Design review of the part built by this model. Coordinates are the model's own, in mm. Face numbers are marked on the shaded views. A direction names the side the tool comes from. Coordinates: 2 decimals unless noted, no trailing zeros. Write each loop counter-clockwise with the first axis right and the second up, starting at its lowest first coordinate (ties: lowest second). Pieces come first, ordered by that corner, then holes. Notation, with made-up numbers: M 87.25,44 L 120.25,44 A19 cw 120.25,65 Z; hole C -38,52.25 d3. An arc over 180 degrees is marked long. Write item = value, one per line.
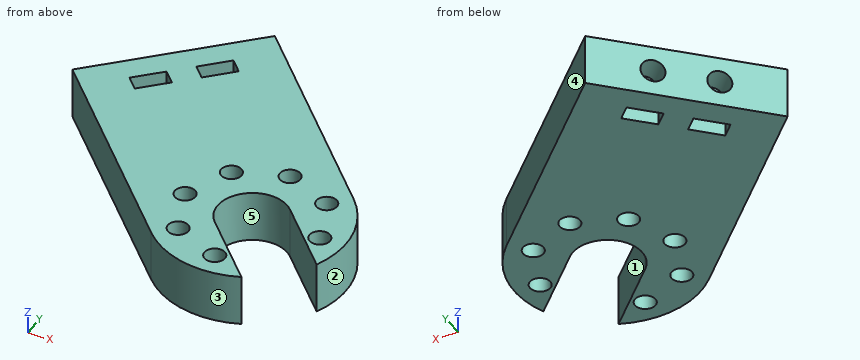
Autodesk Inventor part; units mm, degrees
ref_plane "YZ Plane" through (0, 0, 0) normal (1, 0, 0) x (0, 1, 0)
ref_plane "XZ Plane" through (0, 0, 0) normal (0, 1, 0) x (-1, 0, 0)
ref_plane "XY Plane" through (0, 0, 0) normal (0, 0, 1) x (1, 0, 0)
sketch "스케치1" plane through (0, 0, 0) normal (0, 0, 1) x (1, 0, 0)
  circle A0 centre (-5.6569, -5.6569) radius 1.2
  circle A1 centre (5.6569, -5.6569) radius 1.2
  circle A2 centre (5.6569, 5.6569) radius 1.2
  circle A3 centre (-5.6569, 5.6569) radius 1.2
  circle A4 centre (0, 0) radius 4
  circle A5 centre (0, 0) radius 10.9
  circle A6 centre (0, 8) radius 1.2
  circle A7 centre (8, 0) radius 1.2
  circle A8 centre (0, -8) radius 1.2
  circle A9 centre (-8, 0) radius 1.2
  circle A10 centre (0, 0) radius 4.05
  line L0 (-5.6569, -5.6569) -> (5.6569, 5.6569)
  line L1 (-2.8638, -2.8638) -> (2.8638, 2.8638)
  line L2 (2.8638, 2.8638) -> (13.4704, -7.7428)
  line L3 (13.4704, -7.7428) -> (7.7428, -13.4704)
  line L4 (7.7428, -13.4704) -> (-2.8638, -2.8638)
  line L5 (-5.6569, -5.6569) -> (-8.1671, -8.1671)
  line L6 (5.6569, 5.6569) -> (8.1671, 8.1671)
  line L7 (-7.7075, -7.7075) -> (7.7075, 7.7075)
  line L8 (7.7075, 7.7075) -> (-13.5057, 28.9207)
  line L9 (-13.5057, 28.9207) -> (-28.9207, 13.5057)
  line L10 (-28.9207, 13.5057) -> (-7.7075, -7.7075)
  point P0 (0, 0)
  point P1 (10.0195, -4.2919)
  point P2 (4.2919, -10.0195)
  dimension "d0" = 8.1
  dimension "d1" = 15
  dimension "d2" = 30
extrude "돌출1" add sketch "스케치1" along normal blind 6 contours A0 L0 L4 A5 L5 | A0 L5 A5 L6 A2 L0 A10 | L10 L9 L8 A5 | L0 A2 L6 A5 L2
sketch "스케치4" plane through (-28.9207, 13.5057, 0) normal (-0.7071, 0.7071, 0) x (-0.7071, -0.7071, 0)
  line L0 (0, 6) -> (-7.3, 6)
  line L1 (-21.8, 6) -> (0, 6)
  line L2 (-21.8, 0) -> (0, 0)
  line L3 (0, 0) -> (0, 6)
  line L4 (-21.8, 6) -> (0, 6)
  line L5 (-21.8, 0) -> (-21.8, 6)
  line L6 (-21.8, 0) -> (-14.5, 0)
  line L7 (-14.5, 0) -> (-14.5, 6)
  line L8 (-14.5, 0) -> (-14.5, 6)
  line L9 (-14.5, 6) -> (-7.3, 6)
  line L10 (-7.3, 6) -> (-7.3, 0)
  line L11 (-7.3, 0) -> (-14.5, 0)
  line L12 (-14.5, 6) -> (-14.5, 3)
  line L13 (-7.3, 3) -> (-14.5, 3)
  circle A0 centre (-7.3, 3) radius 1.35
  circle A1 centre (-14.5, 3) radius 1.35
  point P0 (-10.9, 0)
  dimension "d19" = 7.3
  dimension "d20" = 2.7
  dimension "d21" = 2.7
extrude "돌출3" cut sketch "스케치4" against normal blind 4 contours A0 L10 | L10 L13 A0 | A1 L13 L7 | L7 A1 | L10 A0 L13 | L13 A1 L7
sketch "스케치5" plane through (0, 0, 6) normal (0, 0, 1) x (1, 0, 0)
  line L0 (-21.885, 14.8846) -> (-19.9758, 16.7938)
  line L1 (-16.7938, 19.9758) -> (-14.8846, 21.885)
  line L2 (-18.809, 16.5463) -> (-20.2233, 17.9605)
  line L3 (-20.2233, 17.9605) -> (-23.0517, 15.1321)
  line L4 (-23.0517, 15.1321) -> (-21.6375, 13.7179)
  line L5 (-21.6375, 13.7179) -> (-18.809, 16.5463)
  line L6 (-18.809, 16.5463) -> (-23.0517, 15.1321) construction
  line L7 (-20.2233, 17.9605) -> (-21.6375, 13.7179) construction
  line L8 (-13.7179, 21.6375) -> (-15.1321, 23.0517)
  line L9 (-15.1321, 23.0517) -> (-17.9605, 20.2233)
  line L10 (-17.9605, 20.2233) -> (-16.5463, 18.809)
  line L11 (-16.5463, 18.809) -> (-13.7179, 21.6375)
  line L12 (-13.7179, 21.6375) -> (-17.9605, 20.2233) construction
  line L13 (-15.1321, 23.0517) -> (-16.5463, 18.809) construction
  point P0 (0, 0)
  point P1 (-20.9304, 15.8392)
  point P2 (-15.8392, 20.9304)
  dimension "d24" = 2
  dimension "d25" = 4
  dimension "d26" = 2
  dimension "d27" = 4
extrude "돌출4" cut sketch "스케치5" against normal blind 6
properties part number "_armpit_adt_1" material "PMMA 플라스틱"
Q1. For P1, Ø2, axis at y = -1.5, z = 1, coming from the +X side; P2, Ø2, axis at x = 1.5, z = 3, coming from the -Y side; P3, Ø3, axis at x = -17, z = 5, coming from the -Y side (3 decimals), all flat-tipped, find the tip position at first contact; note any pin that passes through.
Check result:
P1 = 10.89
P2 = -10.89
P3 = 0.085
Q2. Wall thickness on line 1 (Y direction, x = 0, z = 2.55) (3 decimals); line 2 (Y direction, x = 1, z = 4.7) (3 decimals); line 3 (Y direction, x = -8, z = 4.1) (3 decimals): over which ranges is each line inside the solid? List them lowest first.
Check result:
line_1 = -10.9 to -9.2, -6.8 to -5.728, 4.05 to 6.8, 9.2 to 15.415
line_2 = -10.854 to -8.663, -7.337 to -6.728, 3.925 to 7.337, 8.663 to 14.415
line_3 = -7.415 to -1.2, 1.2 to 23.415
Q3. The part is to be moulded in two halves that separate along Y. For the marked faces 3, 4 and 5, say which applies: +Y half, -Y half, draft (parallel to the pull), parting line (faces both ways), or undercut.
Check result:
face_3 = -Y half
face_4 = +Y half
face_5 = undercut
Q4. Consider section C-C, the plane x = 0. State the section outline as (y, z) points (3 decimals).
Check result:
outline = M -10.9,0 L -9.2,0 L -9.2,6 L -10.9,6 Z; M -6.8,0 L -5.728,0 L -5.728,6 L -6.8,6 Z; M 4.05,0 L 6.8,0 L 6.8,6 L 4.05,6 Z; M 9.2,0 L 15.415,0 L 15.415,6 L 9.2,6 Z
Q5. Machinability: for the marked faces 1 and 2, which of the approach directions +Z, -Z, +X, -X, +Y, -Y give a long, thin tool a straight path to every point of the face, cutting with its end or side? Answer none if there is none.
Check result:
face_1 = +Z, -Z
face_2 = +Z, -Z, +X
Q6. Consider section A-A, the plane x = -8.5. State the section outline as (y, z) points (3 decimals), and give its area (3 significant figures).
Check result:
outline = M -6.915,0 L -1.091,0 L -1.091,6 L -6.915,6 Z; M 1.091,0 L 23.915,0 L 23.915,6 L 1.091,6 Z
area = 172 mm²
Q7. Consider section B-B, the plane z = 5. State how many separate pieces and enclosed holes the cut face has, and give its area (3 significant figures).
Check result:
separate_pieces = 1
enclosed_holes = 9
area = 681 mm²
